Can you work these out from the model? Positions are in its coordinate system, mm. A direction names the side the tool comes from. Give positions to 0.01 mm unless a question says otherwise; leave off trailing zeros. Write each loop counter-clockwise with the first axis right and the second up, starting at its lowest first coordinate (ties: lowest second). Pieces come first, ordered by that corner, then holes.
from build123d import *
from build123d.topology import SkipClean

# Parameters (mm, degrees)
BOSS_EXTRUDE1_DEPTH = 3
SKETCH2_R           = 1.35
CUT_EXTRUDE1_DEPTH  = 27.795522014
SKETCH3_R           = 2.5
CUT_EXTRUDE2_DEPTH  = 2
SKETCH4_W           = 3
SKETCH4_H           = 30
BOSS_EXTRUDE2_DEPTH = 35
SKETCH5_R           = 1.1
CUT_EXTRUDE3_DEPTH  = 47.400431032
SKETCH6_W           = 13
SKETCH6_H           = 20
CUT_EXTRUDE4_DEPTH  = 47.400431032
CHAMFER1_SIZE       = 10
CHAMFER2_SIZE       = 1
CHAMFER3_SIZE       = 3
SKETCH7_R           = 2
CUT_EXTRUDE5_DEPTH  = 2
CUT_EXTRUDE6_DEPTH  = 0.2
SKETCH9_W           = 2.2
SKETCH9_H           = 2.2
CUT_EXTRUDE7_DEPTH  = 0.2


with BuildPart() as part:
    # Sketch1 → Boss-Extrude1 (new body)
    with BuildSketch(Plane(origin=(0, 0, 0), x_dir=(1, 0, 0), z_dir=(0, 1, 0))):
        Polygon((0, -22), (0, 22), (15, 22), (15, 15), (8, 15), (8, -15), (15, -15), (15, -22), align=None)
    extrude(amount=BOSS_EXTRUDE1_DEPTH)

    # Sketch2 → Cut-Extrude1 (cut, through all)
    with BuildSketch(Plane(origin=(0, 3, 0), x_dir=(1, 0, 0), z_dir=(0, 1, 0))):
        with Locations(Location((10.5, 18.5, 0), (0, 0, 270))):
            Circle(SKETCH2_R)
        with Locations(Location((10.5, -18.5, 0), (0, 0, 270))):
            Circle(SKETCH2_R)
    extrude(amount=-CUT_EXTRUDE1_DEPTH, mode=Mode.SUBTRACT)

    # Sketch3 → Cut-Extrude2 (cut)
    with BuildSketch(Plane(origin=(0, 3, 0), x_dir=(1, 0, 0), z_dir=(0, 1, 0))):
        with Locations(Location((10.5, 18.5, 0), (0, 0, 270))):
            Circle(SKETCH3_R)
        with Locations(Location((10.5, -18.5, 0), (0, 0, 270))):
            Circle(SKETCH3_R)
    extrude(amount=-CUT_EXTRUDE2_DEPTH, mode=Mode.SUBTRACT)

    # Sketch4 → Boss-Extrude2 (add)
    with BuildSketch(Plane(origin=(0, 3, 0), x_dir=(1, 0, 0), z_dir=(0, 1, 0))):
        with Locations((1.5, 0)):
            Rectangle(SKETCH4_W, SKETCH4_H)
    extrude(amount=BOSS_EXTRUDE2_DEPTH)

    # Sketch5 → Cut-Extrude3 (cut, through all)
    with BuildSketch(Plane.ZY):
        with Locations((-10.5, 34.5)):
            Circle(SKETCH5_R)
        with Locations((10.5, 34.5)):
            Circle(SKETCH5_R)
        with Locations((10.5, 22)):
            Circle(SKETCH5_R)
        with Locations((-10.5, 22)):
            Circle(SKETCH5_R)
    extrude(amount=-CUT_EXTRUDE3_DEPTH, mode=Mode.SUBTRACT)

    # Sketch6 → Cut-Extrude4 (cut, through all)
    with BuildSketch(Plane.ZY):
        with Locations((0, 25)):
            Rectangle(SKETCH6_W, SKETCH6_H)
    extrude(amount=-CUT_EXTRUDE4_DEPTH, mode=Mode.SUBTRACT)

    # Chamfer1
    # the kernel refuses this chamfer: 10 mm, written as the material it adds along each edge
    with BuildSketch(Plane(origin=(0, 3, -15), x_dir=(0, -0.02749587661058636, -0.9996219169112968), z_dir=(1, 0, 0))) as chamfer1_piece_1_section:
        Polygon((CHAMFER1_SIZE * 0.999621916911, CHAMFER1_SIZE * 0.0274958766106), (-CHAMFER1_SIZE * 0.0274958766106, CHAMFER1_SIZE * 0.999621916911), (0, 0), align=None)
    chamfer1_piece_1 = extrude(amount=3, mode=Mode.PRIVATE)
    chamfer1_piece_1 = split(chamfer1_piece_1, bisect_by=Plane(origin=(1.5, 6.564102564, -22), z_dir=(0, 0, 1)), keep=Keep.TOP, mode=Mode.PRIVATE)
    add(chamfer1_piece_1)
    with BuildSketch(Plane(origin=(3, 3, 15), x_dir=(0, -0.02749587661058636, 0.9996219169112968), z_dir=(-1, 0, 0))) as chamfer1_piece_2_section:
        Polygon((CHAMFER1_SIZE * 0.999621916911, CHAMFER1_SIZE * 0.0274958766106), (-CHAMFER1_SIZE * 0.0274958766106, CHAMFER1_SIZE * 0.999621916911), (0, 0), align=None)
    chamfer1_piece_2 = extrude(amount=3, mode=Mode.PRIVATE)
    chamfer1_piece_2 = split(chamfer1_piece_2, bisect_by=Plane(origin=(1.5, 6.564102564, 22), z_dir=(0, 0, -1)), keep=Keep.TOP, mode=Mode.PRIVATE)
    add(chamfer1_piece_2)

    # Chamfer2
    chamfer2_edges = [part.edges().sort_by_distance(p)[0] for p in [
        (0, 25, -6.5),
        (0, 15, 0),
        (0, 25, 6.5),
        (0, 35, 0),
    ]]
    chamfer(chamfer2_edges, length=CHAMFER2_SIZE)

    # Chamfer3
    chamfer3_edges = [part.edges().sort_by_distance(p)[0] for p in [
        (1.5, 38, 15),
        (1.5, 38, -15),
    ]]
    chamfer(chamfer3_edges, length=CHAMFER3_SIZE)

    # Sketch7 → Cut-Extrude5 (cut)
    with BuildSketch(Plane.ZY):
        with Locations((-10.5, 34.5)):
            Circle(SKETCH7_R)
        with Locations((10.5, 34.5)):
            Circle(SKETCH7_R)
        with Locations((10.5, 22)):
            Circle(SKETCH7_R)
        with Locations((-10.5, 22)):
            Circle(SKETCH7_R)
    extrude(amount=-CUT_EXTRUDE5_DEPTH, mode=Mode.SUBTRACT)

    # Sketch8 → Cut-Extrude6 (cut)
    with SkipClean():  # the faces are left unmerged after this step: merging them gives an invalid solid
        with BuildSketch(Plane.ZY.offset(-2)):
            with BuildLine():
                Line((-11.6, 32.829670691), (-11.6, 36.170329309))
                ThreePointArc((-11.6, 36.170329309), (-10.5, 36.5), (-9.4, 36.170329309))
                Line((-9.4, 36.170329309), (-9.4, 32.829670691))
                ThreePointArc((-9.4, 32.829670691), (-10.5, 32.5), (-11.6, 32.829670691))
            make_face()
            with BuildLine():
                Line((-11.6, 20.329670691), (-11.6, 23.670329309))
                ThreePointArc((-11.6, 23.670329309), (-10.5, 24), (-9.4, 23.670329309))
                Line((-9.4, 23.670329309), (-9.4, 20.329670691))
                ThreePointArc((-9.4, 20.329670691), (-10.5, 20), (-11.6, 20.329670691))
            make_face()
        cut_extrude6 = extrude(amount=-CUT_EXTRUDE6_DEPTH, mode=Mode.SUBTRACT)

    # Sketch9 → Cut-Extrude7 (cut)
    with SkipClean():  # the faces are left unmerged after this step: merging them gives an invalid solid
        with BuildSketch(Plane.ZY.offset(-2.2)):
            with Locations((-10.5, 22)):
                Rectangle(SKETCH9_W, SKETCH9_H)
            with Locations((-10.5, 34.5)):
                Rectangle(SKETCH9_W, SKETCH9_H)
        cut_extrude7 = extrude(amount=-CUT_EXTRUDE7_DEPTH, mode=Mode.SUBTRACT)

    # Mirror1: Cut-Extrude6, Cut-Extrude7 across plane
    with SkipClean():  # the faces are left unmerged after this step: merging them gives an invalid solid
        add(cut_extrude6.mirror(Plane.XY), mode=Mode.SUBTRACT)
        add(cut_extrude7.mirror(Plane.XY), mode=Mode.SUBTRACT)


solid = part.part
(1) Imagine slicing it at B-B, the plane z = 4. Write out the boundary of the cut face in (x, y), plus the area to 3 significant figures.
Returned:
outline: (0, 0) - (8, 0) - (8, 3) - (3, 3) - (3, 15) - (1, 15) - (0, 14) - close; (0, 36) - (1, 35) - (3, 35) - (3, 38) - (0, 38) - close
area: 68.0 mm2
(2) If we mould it in two halves opening along Y, with no side actions, what happens to faces 6 (the face through (2.7, 35.43, 11.09)), 7 (the face through (1, 9, -19)), 8 (the face through (6, 2, 22))? For each: +Y half, -Y half, draft (parallel to the pull), parting line (faces both ways), or undercut.
Returned:
face 6: undercut
face 7: +Y half
face 8: draft
(3) Will these pins go through, and if not, where does the flat tip stop? P1, Ø5.5, axis at x = 11, z = 19, coming from the +Y side; P2, Ø3, axis at y = 22, z = -10.5, coming from the +X side; P3, Ø1, axis at x = 2.5, y = 25.5, coming from the +Z side.
Returned:
P1: stops at y = 3
P2: stops at x = 3
P3: stops at z = 15
(4) For faces 1 (the face through (0.5, 24.8, -7)), 2 (the face through (6, 0, 0)), 3 (the face through (8, 1, 0)), 4 (the face through (1, 24, -15)), 5 (the face through (9, 2, 16.5)), which set-ups out of +Z, -Z, +X, -X, +Y, -Y let a thin tool reach every point of the face, with its end or its side?
Returned:
face 1: -X
face 2: +Z, -Z, +X, -X, -Y
face 3: +X, +Y, -Y
face 4: -Z, +X, -X, +Y
face 5: +Y
(5) If I drill on L1, parallel to Z at x = 1, y = 22; L2, parallel to Y at x = 0.8, z = 10.5; L3, parallel to Y at x = 2.85, z = -10.5, over which ranges is the centre line in solid material (lowest first)?
Returned:
L1: z = -15 to -12.5, -8.5 to -6.5, 6.5 to 8.5, 12.5 to 15
L2: y = 0 to 20, 24 to 32.5, 36.5 to 38
L3: y = 0 to 20.9, 23.1 to 33.4, 35.6 to 38
(6) Imagine slicing it at C-C, the plane x = 10.5. Write out the boundary of the cut face in (y, z).
Returned:
outline: (0, -22) - (3, -22) - (3, -21) - (1, -21) - (1, -19.85) - (0, -19.85) - close; (0, -17.15) - (1, -17.15) - (1, -16) - (3, -16) - (3, -15) - (0, -15) - close; (0, 15) - (3, 15) - (3, 16) - (1, 16) - (1, 17.15) - (0, 17.15) - close; (0, 19.85) - (1, 19.85) - (1, 21) - (3, 21) - (3, 22) - (0, 22) - close
(7) Imagine slicing it at D-D, the plane z = -18.5. Write out the boundary of the cut face in (x, y).
Returned:
outline: (0, 0) - (9.15, 0) - (9.15, 1) - (8, 1) - (8, 3) - (3, 3) - (3, 9.5) - (0, 9.5) - close; (11.85, 0) - (15, 0) - (15, 3) - (13, 3) - (13, 1) - (11.85, 1) - close
(8) Imagine slicing it at A-A, the plane x = 14.25. Write out the boundary of the cut face in (y, z), plus the area to 3 significant figures.
Returned:
outline: (0, -22) - (3, -22) - (3, -15) - (0, -15) - close; (0, 15) - (3, 15) - (3, 22) - (0, 22) - close
area: 42.0 mm2
